The figure shows three views and two pictorial views of one solid part (mm, origin at its lowest corner). Answer the questions. A direction names the side the tool comes from. Coordinates: 2 decimals unless noted, no trailing zeros. Loops run counter-clockwise (first coordinate to the right, second up) from the corner with the lowest first, then second, coordinate; pieces in that order, holes last. Notation, with made-up numbers: (87, 44.5) -> (121, 44.5) arc R16 cw to (121, 68.5) -> close; hole circle Ø2 at (24.25, 9.25). An arc over 180 degrees is marked (long way). Use a Markdown table: item, result. Add a question column.
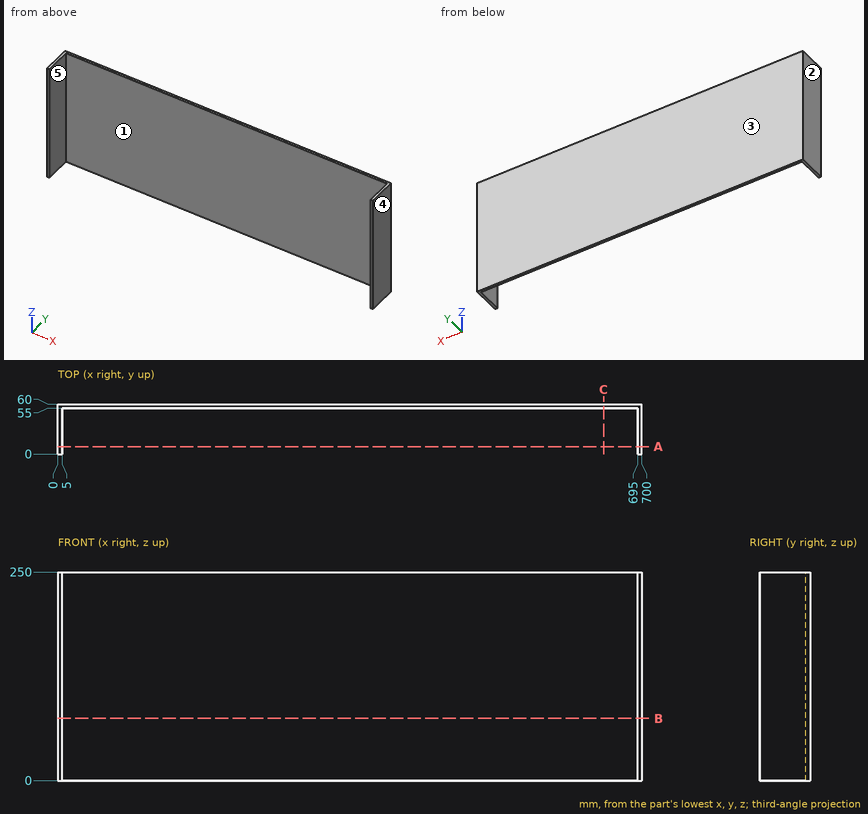
Item 1: For a pull along X with two mould halves and no side action, classify the marked faces 1, 2 and 3 as +X half, -X half, draft (parallel to the pull), parting line (faces both ways), or undercut.
Item 2: Section C-C (x = 654) is taken. Determine the outline of the cut face in (y, z).
Item 3: Find the intervals of material crossed by probe 1 along X at (y, z) = (48, 143.5); probe 2 along Y at (x, z) = (245, 93), in increasing order.
Item 4: Section B-B (z = 74.5) is taken. Determine the outline of the cut face in (x, y), then the cut area to 3 significant figures.
Item 5: For the marked faces 4 and 5, determine the directions among +Z, -Z, +X, -X, +Y, -Y from which every point of the face is accessible in a straight line to the end or side of a thin tool.
Item 6: Given pin 1 (5 mm diameter, centred on x = 477, z = 154.5, fed in from -Y), flat-ended and moving along its own axis, determine where the tip first touches the part or whether it passes through.
Item 7: Section A-A (y = 9) is taken. Determine the outline of the cut face in (x, z), then the cut area to 3 significant figures.
Output:
| question | item | result |
|---|---|---|
| 1 | face 1 | undercut |
| 1 | face 2 | -X half |
| 1 | face 3 | draft |
| 2 | outline | (55, 0) -> (60, 0) -> (60, 250) -> (55, 250) -> close |
| 3 | probe 1 | x = 0 to 5, 695 to 700 |
| 3 | probe 2 | y = 55 to 60 |
| 4 | outline | (0, 0) -> (5, 0) -> (5, 55) -> (695, 55) -> (695, 0) -> (700, 0) -> (700, 60) -> (0, 60) -> close |
| 4 | area | 4,050 mm2 |
| 5 | face 4 | +Z, -Z, +X, +Y, -Y |
| 5 | face 5 | +Z, -Z, -Y |
| 6 | pin 1 | stops at y = 55 |
| 7 | outline | (0, 0) -> (5, 0) -> (5, 250) -> (0, 250) -> close; (695, 0) -> (700, 0) -> (700, 250) -> (695, 250) -> close |
| 7 | area | 2,500 mm2 |
